Geometry check sheet. Reference: the model listing, model coordinates, mm. A direction names the side the tool comes from. Give positions to 0.01 mm unless a question says otherwise; leave off trailing zeros. Write each loop counter-clockwise with the first axis right and the second up, starting at its lowest first coordinate (ties: lowest second). Pieces come first, ordered by that corner, then holes. Notation, with made-up numbers: (42, 79.25) -> (48, 79.25) arc R19 cw to (48, 106.25) -> close; hole circle Ø1 at (82.25, 84.5). An arc over 180 degrees is marked (long way). One line per item, written item: value.
Autodesk Inventor part; units mm, degrees
ref_plane "YZ Plane" through (0, 0, 0) normal (1, 0, 0) x (0, 1, 0)
ref_plane "XZ Plane" through (0, 0, 0) normal (0, 1, 0) x (-1, 0, 0)
ref_plane "XY Plane" through (0, 0, 0) normal (0, 0, 1) x (1, 0, 0)
sketch "Sketch1" plane through (0, 0, 0) normal (0, 1, 0) x (-1, 0, 0)
  line L0 (0, 0) -> (0, 56.5412)
  line L1 (5.8682, 61.4653) -> (14.7704, 59.8956)
  line L2 (24.4547, 40.4718) -> (8.4899, 9.1391)
  line L3 (7.4, 4.5992) -> (7.4, 0)
  line L4 (7.4, 0) -> (0, 0)
  line L5 (3.5, 56.5412) -> (3.5, 32.047)
  line L6 (14.846, 29.3231) -> (21.3362, 42.0608)
  line L7 (14.1626, 56.4488) -> (5.2605, 58.0184)
  arc A0 (3.5, 32.047) -> (14.846, 29.3231) centre (9.5, 32.047) ccw
  arc A1 (5.2605, 58.0184) -> (3.5, 56.5412) centre (5, 56.5412) ccw
  arc A2 (5.8682, 61.4653) -> (0, 56.5412) centre (5, 56.5412) ccw
  arc A3 (21.3362, 42.0608) -> (14.1626, 56.4488) centre (12.4261, 46.6007) ccw
  arc A4 (24.4547, 40.4718) -> (14.7704, 59.8956) centre (12.4261, 46.6007) ccw
  arc A5 (8.4899, 9.1391) -> (7.4, 4.5992) centre (17.4, 4.5992) ccw
  point P0 (0, 62.5)
  point P1 (7.4, 7)
  dimension "d0" = 7.4
  dimension "d5" = 27
  dimension "d6" = 80
  dimension "d7" = 7
  dimension "d8" = 6
  dimension "d9" = 1.5
  dimension "d10" = 62.5
  dimension "d12" = 3.5
  dimension "d13" = 10
  dimension "d15" = 10
extrude "Extrusion1" add sketch "Sketch1" along normal blind 3
fillet "Fillet1" radius 0.5 13 edges at (-3.5, 3, 44.2941) (-4.0358, 3, 57.6903) (-9.7116, 3, 57.2336) (-21.3755, 3, 51.0627) (-18.0911, 3, 35.6919) (-8.0993, 3, 26.2128) (-1.7861, 3, 60.3715) (-10.3193, 3, 60.6804) (-24.5078, 3, 52.6243) (-16.4723, 3, 24.8055) (-7.6763, 3, 6.9337) (-7.4, 3, 2.2996) (0, 3, 28.2706)
sketch "Sketch2" plane through (0, 0, 0) normal (0, -1, 0) x (1, 0, 0)
  line L0 (0, 0) -> (0, 56.5412)
  line L1 (-7.4, 0) -> (0, 0)
  line L2 (0, 52.2) -> (1.25, 52.2)
  line L3 (1.25, 52.2) -> (1.25, 47)
  line L4 (1.25, 47) -> (0, 47)
  dimension "d19" = 1.25
  dimension "d20" = 5.2
  dimension "d21" = 47
extrude "Extrusion2" add sketch "Sketch2" against normal blind 2
fillet "Fillet2" radius 0.5 8 edges at (1.25, 2, 49.6) (1.25, 1, 52.2) (0.625, 2, 52.2) (0.625, 2, 47) (1.25, 1, 47) (0, 1, 52.2) (0, 2, 49.6) (0, 1, 47)
properties part number "Agarre tijeras (mitad 1)"
1) Mould release check, pull along X, two halves, no side actions. Record for faces 1 (the flat face through (-4, 1, 0)), 2 (the cylindrical face through (-16.45, 2.857, 25.093)), 3 (the flat face through (0, 1, 28)), 4 (the cylindrical face through (-8.209, 1.232, 26.188)): released by +X, released by -X, zero draft, split by the parting line, or undercut.
Verdict:
face 1: zero draft
face 2: released by -X
face 3: released by +X
face 4: undercut
2) Depth check by flat-ended pin: pin 1 Ø1.2 at (y, z) = (1.5, 44.5) entering from -X; pin 2 Ø3 at (x, z) = (-14.5, 16.5) entering from -Y. Enter the tip coordinate at first touch or a pass-through.
Verdict:
pin 1: x = -25.84
pin 2: through
3) Sectioned sample at A-A on y = 1.05. Record the cut outline in (x, z).
Verdict:
outline: (-24.45, 40.47) -> (-8.49, 9.14) arc R10 cw to (-7.4, 4.6) -> (-7.4, 0) -> (0, 0) -> (0, 46.5) arc R0.5 cw to (0.5, 47) -> (0.75, 47) arc R0.5 ccw to (1.25, 47.5) -> (1.25, 51.7) arc R0.5 ccw to (0.75, 52.2) -> (0.5, 52.2) arc R0.5 cw to (0, 52.7) -> (0, 56.54) arc R5 ccw to (-5.87, 61.47) -> (-14.77, 59.9) arc R13.5 ccw to start; hole (-21.34, 42.06) -> (-14.85, 29.32) arc R6 ccw to (-3.5, 32.05) -> (-3.5, 56.54) arc R1.5 ccw to (-5.26, 58.02) -> (-14.16, 56.45) arc R10 ccw to start
4) Tool access check on faces 5 (the cylindrical face through (-9.674, 2.85, 57.385)), 6 (the flat face through (-3, 0, 31)), 7 (the cylindrical face through (-21.316, 1.232, 51.179)). Record the directions out of +Z, -Z, +X, -X, +Y, -Y that give a thin tool (end or side, any length) a straight path to the whole face; none if there is none.
Verdict:
face 5: +Y
face 6: +Z, -Z, +X, -X, -Y
face 7: +Y, -Y
5) Scan lines: probe 1 along Z at (x, y) = (-18.5, 0.75); probe 2 along Z at (x, y) = (-21.5, 0.65); probe 3 along X at (y, z) = (1.4, 36). Record each from-to range of solid material in increasing order.
Verdict:
probe 1: 28.79 to 36.49, 54.54 to 58.66
probe 2: 34.67 to 42.4, 50.8 to 56.6
probe 3: -22.18 to -18.25, -3.5 to 0
